Source: three-view drawing plus pictorial views. Frame: mm from the lowest corner of the part. Give positions to 0.01 mm unless a question says otherwise; leave off trailing zeros. Loops run counter-clockwise (first coordinate to the right, second up) from the corner with the lowest first, then second, coordinate; pieces in that order, holes last. Notation, with made-up numbers: (-8.75, -13) - (35.25, -13) arc R20 cw to (35.25, -4) - close; hole circle Ø7 at (30, -17.75). An arc over 180 degrees is marked (long way). Answer in a Markdown table with one row per item.
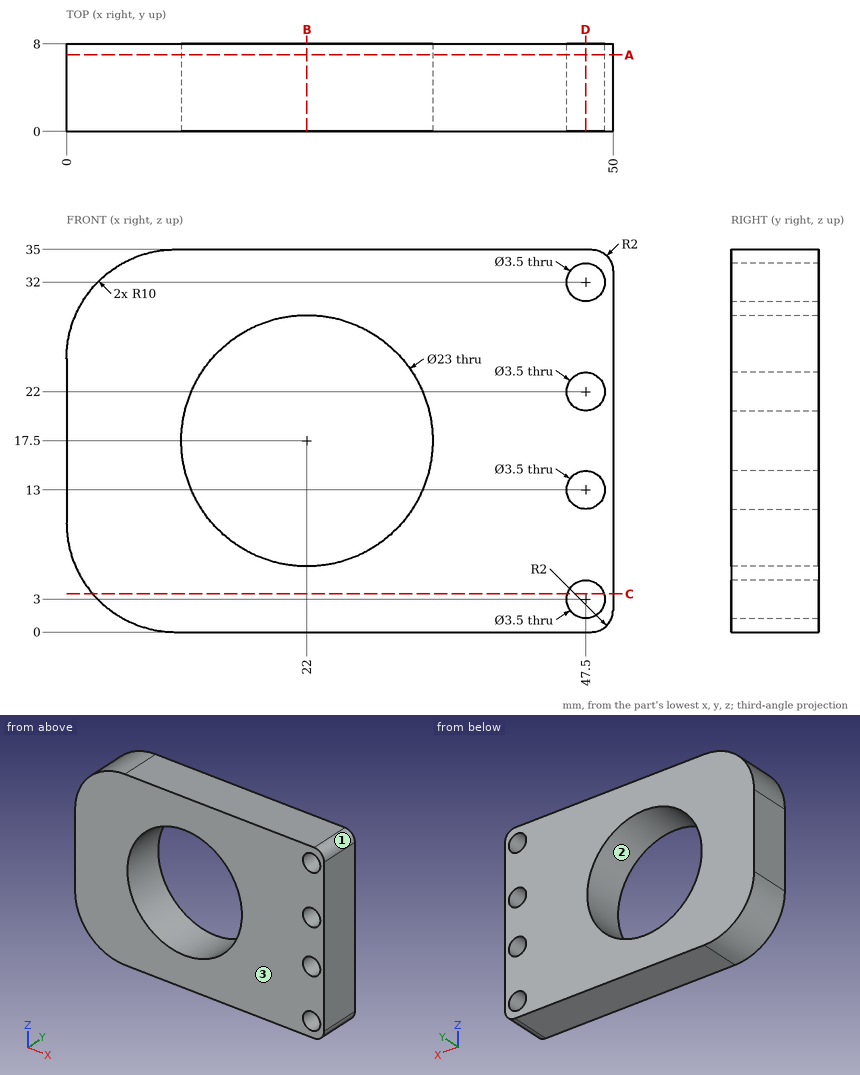
Q1. Cut plane C-C (z = 3.5). Output: boundary loops of the cut face in (x, y).
Check values:
| item | result |
|---|---|
| outline | (2.4, 0) - (45.82, 0) - (45.82, 8) - (2.4, 8) - close; (49.18, 0) - (50, 0) - (50, 8) - (49.18, 8) - close |
Q2. Draft query along Z for the marked faces 1, 2 and 3. Return one class per face: pulls with the +Z half, pulls with the -Z half, needs draft (parallel to the pull), parting line crosses it, or undercut.
Check values:
| item | result |
|---|---|
| face 1 | pulls with the +Z half |
| face 2 | undercut |
| face 3 | needs draft |
Q3. Material intervals for line 1 along X through (y, z) = (5.75, 14.5); line 2 along X through (y, z) = (3, 3); line 3 along X through (y, z) = (3, 13), sorted ascending.
Check values:
| item | result |
|---|---|
| line 1 | 0 to 10.9, 33.1 to 46.6, 48.4 to 50 |
| line 2 | 2.86 to 45.75, 49.25 to 50 |
| line 3 | 0 to 11.42, 32.58 to 45.75, 49.25 to 50 |
Q4. Cut plane B-B (x = 22). Output: boundary loops of the cut face in (y, z).
Check values:
| item | result |
|---|---|
| outline | (0, 0) - (8, 0) - (8, 6) - (0, 6) - close; (0, 29) - (8, 29) - (8, 35) - (0, 35) - close |
Q5. Cut plane D-D (x = 47.5). Output: boundary loops of the cut face in (y, z).
Check values:
| item | result |
|---|---|
| outline | (0, 0) - (8, 0) - (8, 1.25) - (0, 1.25) - close; (0, 4.75) - (8, 4.75) - (8, 11.25) - (0, 11.25) - close; (0, 14.75) - (8, 14.75) - (8, 20.25) - (0, 20.25) - close; (0, 23.75) - (8, 23.75) - (8, 30.25) - (0, 30.25) - close; (0, 33.75) - (8, 33.75) - (8, 35) - (0, 35) - close |
Q6. Cut plane A-A (y = 7). Output: boundary loops of the cut face in (x, z), and give its area (3 significant figures).
Check values:
| item | result |
|---|---|
| outline | (0, 10) arc R10 ccw to (10, 0) - (48, 0) arc R2 ccw to (50, 2) - (50, 33) arc R2 ccw to (48, 35) - (10, 35) arc R10 ccw to (0, 25) - close; hole circle Ø23 at (22, 17.5); hole circle Ø3.5 at (47.5, 3); hole circle Ø3.5 at (47.5, 13); hole circle Ø3.5 at (47.5, 22); hole circle Ø3.5 at (47.5, 32) |
| area | 1,250 mm² |
